Design review of the part built by this model. Coordinates are the model's own, in mm. Face numbers are marked on the shaded views. Round coordinates to 2 decimals unless told otherwise and drop trailing zeros. Write each loop counter-clockwise with the first axis right and the second up, starting at its lowest first coordinate (ties: lowest second). Pieces come first, ordered by that corner, then holes. Notation, with made-up numbers: (16.25, 11.5) -> (28.25, 11.5) arc R10 ccw to (28.25, 30.5) -> close; hole circle Ø9 at (30, 13). An arc over 180 degrees is marked (long way). Write item = value, one per line. Start each with the question number.
Item 1: Add section D-D, the plane y = 49.5. State the section outline as (x, z) points, then the cut area to 3 significant figures.
Item 2: For pin 1 Ø3 at (x, y) = (-3.5, 33.5) entering from +Z; pin 2 Ø2 at (x, z) = (26, -9.5) entering from +Y; pin 3 Ø2 at (x, y) = (-6.5, 78.5) entering from +Z, all flat-tipped, find the tip position at first contact; note any pin that passes through.
Item 3: Mouldability with a two-part tool opening along Z and no side actions: class the marked faces 1, 2 and 3 as released by +Z, released by -Z, zero draft, split by the parting line, or undercut.
Item 4: Add section A-A, the plane z = 0. State the section outline as (x, y) points.
Item 5: To check wall thickness, follow L1, parallel to X at y = 124, z = 0; L2, parallel to Y at x = -27, z = -8; L3, parallel to X at y = 36.5, z = -38. State the ranges of each line that lie inside material, in increasing order.
Item 6: Add section B-B, the plane y = 127. State the section outline as (x, z) points, then the cut area to 3 significant figures.
Item 7: Add section C-C, the plane x = 0. State the section outline as (y, z) points.
from build123d import *

# Parameters (mm, degrees)
SKETCH_1_R          = 72.25
SKETCH_1_R_2        = 71
EXTRUDE_1_DEPTH     = 140
SKETCH_2_W          = 2
SKETCH_2_H          = 3
CHAMFER_3_SIZE      = 0.803847577
CHAMFER_3_SIZE_2    = 3
CHAMFER_5_SIZE      = 3
CHAMFER_5_SIZE_2    = 0.803847577
SKETCH_3_R          = 62.25
CUT_EXTRUDE_7_DEPTH = 135
CUT_EXTRUDE_START   = 135
SKETCH_8_R          = 69.5
CUT_EXTRUDE_9_DEPTH = 80


with BuildPart() as part:
    # 草圖1 → 填料-伸長1 (new body)
    # profile 1 of 2: a face of its own
    with BuildSketch(Plane(origin=(0, 0, 0), x_dir=(1, 0, 0), z_dir=(0, 1, 0))):
        with Locations(Location((0, 0, 0), (0, 0, 270))):
            Circle(SKETCH_1_R)
        Circle(SKETCH_1_R_2, mode=Mode.SUBTRACT)
    # profile 2 of 2: a face of its own
    with BuildSketch(Plane(origin=(0, 0, 0), x_dir=(1, 0, 0), z_dir=(0, 1, 0))):
        Circle(SKETCH_1_R_2)
    extrude(amount=EXTRUDE_1_DEPTH)

    # 草圖2 → 除料-旋轉1 (revolve, cut)
    with BuildSketch(Plane.XY, mode=Mode.PRIVATE) as cut_revolve_1_sk:
        with Locations((71.25, 5)):
            Rectangle(SKETCH_2_W, SKETCH_2_H)
    revolve(cut_revolve_1_sk.sketch.rotate(Axis((0, 0, 0), (0, 1, 0)), 90), axis=Axis((0, 0, 0), (0, 1, 0)), mode=Mode.SUBTRACT)

    # 導角3
    # the kernel refuses this chamfer: 3, 0.803847577 mm, written as the material it takes off along each edge
    with BuildSketch(Plane(origin=(0, 3.5, 0), x_dir=(0, 0, 1), z_dir=(1, 0, 0))) as chamfer_3_piece_1_section:
        Polygon((72.25, CHAMFER_3_SIZE), (72.25 - CHAMFER_3_SIZE_2, 0), (72.25, 0), align=None)
    chamfer_3_piece_1 = revolve(axis=Axis((0, 3.5, 0), (0, -1, 0)), mode=Mode.PRIVATE)
    chamfer_3_piece_1 = chamfer_3_piece_1 - Plane(origin=(0, 3.028349799, 0), x_dir=(0, 0, -1), z_dir=(0, 1, 0)) * Cylinder(70.25, 289, mode=Mode.PRIVATE)
    add(chamfer_3_piece_1, mode=Mode.SUBTRACT)

    # 導角5
    # the kernel refuses this chamfer: 3, 0.803847577 mm, written as the material it takes off along each edge
    with BuildSketch(Plane(origin=(0, 6.5, 0), x_dir=(0, 0, 1), z_dir=(1, 0, 0))) as chamfer_5_piece_1_section:
        Polygon((72.25 - CHAMFER_5_SIZE, 0), (72.25, -CHAMFER_5_SIZE_2), (72.25, 0), align=None)
    chamfer_5_piece_1 = revolve(axis=Axis((0, 6.5, 0), (0, -1, 0)), mode=Mode.PRIVATE)
    chamfer_5_piece_1 = chamfer_5_piece_1 - Plane(origin=(0, 6.971650201, 0), x_dir=(0, 0, -1), z_dir=(0, 1, 0)) * Cylinder(70.25, 289, mode=Mode.PRIVATE)
    add(chamfer_5_piece_1, mode=Mode.SUBTRACT)

    # 草圖3 → 除料-伸長7 (cut)
    with BuildSketch(Plane(origin=(0, 140, 0), x_dir=(1, 0, 0), z_dir=(0, 1, 0))):
        with Locations(Location((0, 0, 0), (0, 0, 270))):
            Circle(SKETCH_3_R)
    extrude(amount=-CUT_EXTRUDE_7_DEPTH, mode=Mode.SUBTRACT)

    # 草圖8 → 除料-伸長9 (cut)
    with BuildSketch(Plane(origin=(0, 5, 0), x_dir=(1, 0, 0), z_dir=(0, 1, 0)).offset(CUT_EXTRUDE_START)):
        with Locations(Location((0, 0, 0), (0, 0, 270))):
            Circle(SKETCH_8_R)
    extrude(amount=-CUT_EXTRUDE_9_DEPTH, mode=Mode.SUBTRACT)


solid = part.part
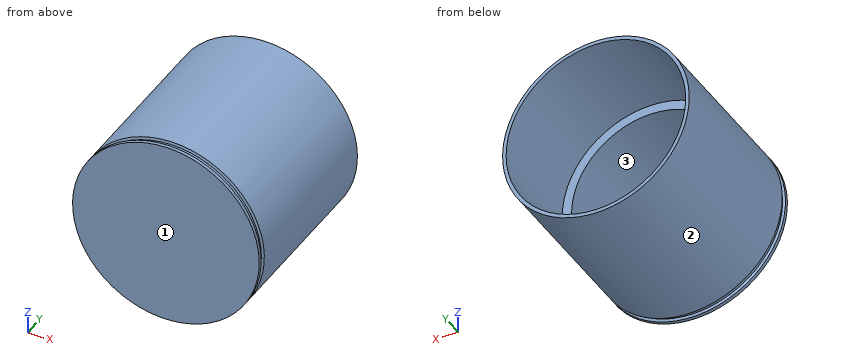
Result set:
q1.outline = circle Ø144.5 at (0, 0); hole circle Ø124.5 at (0, 0)
q1.area = 4,230 mm²
q2.pin_1 = 72.22
q2.pin_2 = 5
q2.pin_3 = 72.04
q3.face_1 = zero draft
q3.face_2 = split by the parting line
q3.face_3 = undercut
q4.outline = (-72.25, 0) -> (72.25, 0) -> (72.25, 2.7) -> (70.25, 3.23) -> (70.25, 6.77) -> (72.25, 7.3) -> (72.25, 140) -> (69.5, 140) -> (69.5, 60) -> (62.25, 60) -> (62.25, 5) -> (-62.25, 5) -> (-62.25, 60) -> (-69.5, 60) -> (-69.5, 140) -> (-72.25, 140) -> (-72.25, 7.3) -> (-70.25, 6.77) -> (-70.25, 3.23) -> (-72.25, 2.7) -> close
q5.L1 = -72.25 to -69.5, 69.5 to 72.25
q5.L2 = 0 to 5
q5.L3 = -61.45 to -49.31, 49.31 to 61.45
q6.outline = circle Ø144.5 at (0, 0); hole circle Ø139 at (0, 0)
q6.area = 1,220 mm²
q7.outline = (0, -72.25) -> (2.7, -72.25) -> (3.23, -70.25) -> (6.77, -70.25) -> (7.3, -72.25) -> (140, -72.25) -> (140, -69.5) -> (60, -69.5) -> (60, -62.25) -> (5, -62.25) -> (5, 62.25) -> (60, 62.25) -> (60, 69.5) -> (140, 69.5) -> (140, 72.25) -> (7.3, 72.25) -> (6.77, 70.25) -> (3.23, 70.25) -> (2.7, 72.25) -> (0, 72.25) -> close
